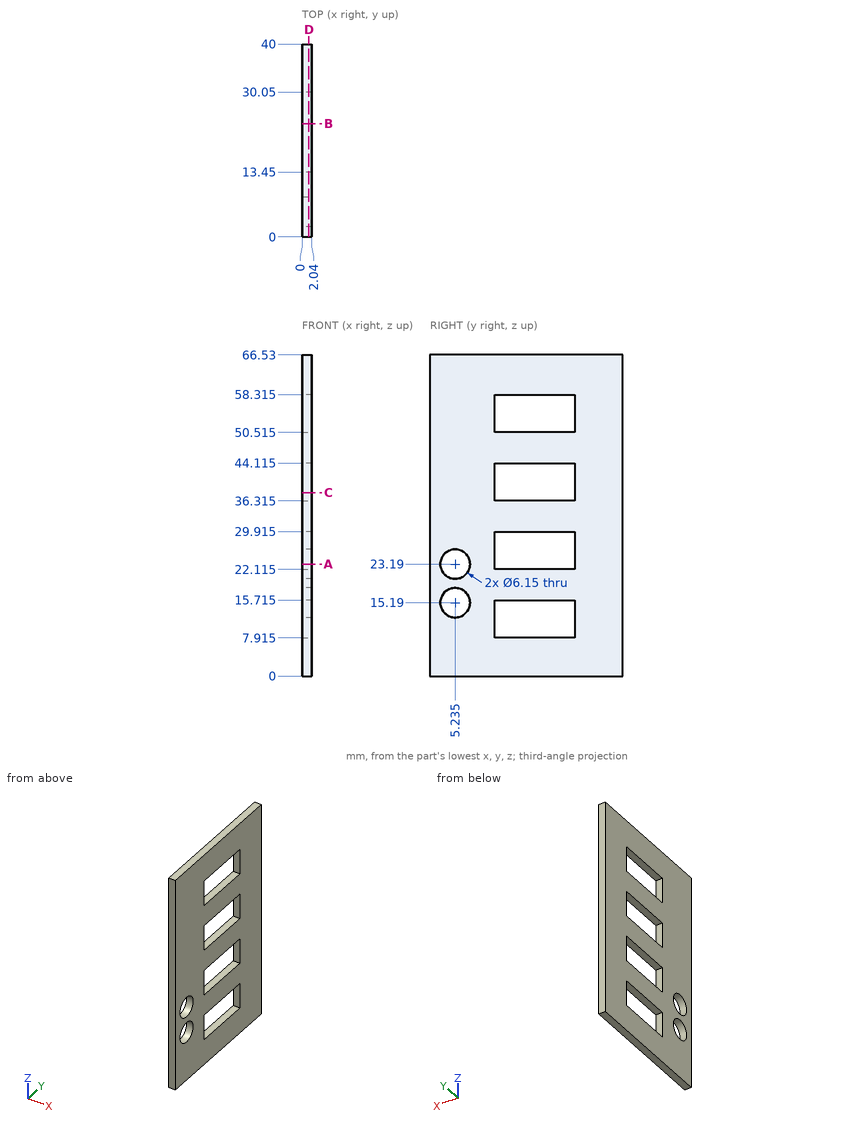
Geometry: see drawing. Coordinates: mm, zero at the bounding-box minimum. Give positions to 0.01 mm unless a question says otherwise; leave off trailing zeros. Order: outer loops, then holes, each group sorted by start corner. A loop starts at its lowest first (then second) coordinate and runs counter-clockwise, first axis right, second up. Notation, with made-up numbers: (38.5, 67) - (74.5, 67) arc R22 cw to (74.5, 100) - close; hole circle Ø7 at (62, 0). An arc over 180 degrees is marked (long way). Use CSV: the item, a comma, the result in double quotes.
1. Section query A-A (z = 23.19). Output: boundary loops of the cut face in (x, y).
Answers below:
outline,"(0, 0) - (2.04, 0) - (2.04, 2.16) - (0, 2.16) - close; (0, 8.31) - (2.04, 8.31) - (2.04, 13.45) - (0, 13.45) - close; (0, 30.05) - (2.04, 30.05) - (2.04, 40) - (0, 40) - close"
2. Section query D-D (x = 1.4). Output: boundary loops of the cut face in (y, z) (3 decimals), plus the area to 3 significant figures.
Answers below:
outline,"(0, 0) - (40, 0) - (40, 66.53) - (0, 66.53) - close; hole circle Ø6.15 at (5.235, 15.19); hole circle Ø6.15 at (5.235, 23.19); hole (13.45, 7.915) - (30.05, 7.915) - (30.05, 15.715) - (13.45, 15.715) - close; hole (13.45, 22.115) - (30.05, 22.115) - (30.05, 29.915) - (13.45, 29.915) - close; hole (13.45, 36.315) - (30.05, 36.315) - (30.05, 44.115) - (13.45, 44.115) - close; hole (13.45, 50.515) - (30.05, 50.515) - (30.05, 58.315) - (13.45, 58.315) - close"
area,"2,080 mm2"
3. Section query C-C (z = 38). Output: boundary loops of the cut face in (x, y), plus the area to 3 significant figures.
Answers below:
outline,"(0, 0) - (2.04, 0) - (2.04, 13.45) - (0, 13.45) - close; (0, 30.05) - (2.04, 30.05) - (2.04, 40) - (0, 40) - close"
area,"47.7 mm2"
4. Section query B-B (y = 23.5). Output: boundary loops of the cut face in (x, z) (3 decimals).
Answers below:
outline,"(0, 0) - (2.04, 0) - (2.04, 7.915) - (0, 7.915) - close; (0, 15.715) - (2.04, 15.715) - (2.04, 22.115) - (0, 22.115) - close; (0, 29.915) - (2.04, 29.915) - (2.04, 36.315) - (0, 36.315) - close; (0, 44.115) - (2.04, 44.115) - (2.04, 50.515) - (0, 50.515) - close; (0, 58.315) - (2.04, 58.315) - (2.04, 66.53) - (0, 66.53) - close"
5. Material intervals for line 1 along Z through (x, y) = (1.1, 18.5) (3 decimals); line 2 along Z through (x, y) = (0.55, 5); line 3 along Y through (x, z) = (1, 15.19), sorted ascending. Write a range as from..to.
Answers below:
line 1,"0..7.915, 15.715..22.115, 29.915..36.315, 44.115..50.515, 58.315..66.53"
line 2,"0..12.12, 18.26..20.12, 26.26..66.53"
line 3,"0..2.16, 8.31..13.45, 30.05..40"
